Check sheet for the modelled part. Datum: model origin and axes. Units: mm. A direction names the side the tool comes from. Coordinates: 2 decimals unless noted, no trailing zeros. Order: outer loops, then holes, each group sorted by start corner. A loop starts at its lowest first (then second) coordinate and runs counter-clockwise, first axis right, second up.
from build123d import *

# Parameters (mm, degrees)
F1_DEPTH     = 113.387234509
F3_DEPTH     = 464.7335410118
F5_DEPTH     = 66.4555206895
F6_R         = 30.48
F8_DEPTH     = 322.3102986813
F10_DEPTH    = 342.2025442123
F12_DEPTH    = 991.1689758301
F13_T4_DEPTH = 1291.048119331


# Not quite as in the source:
# - a fillet or chamfer that OpenCascade refuses, or shapes differently, is made with other operations: its cross-section is extruded or revolved along the edge and cut away or added


with BuildPart() as f1:
    # F0 (on Front) → F1 (new body)
    with BuildSketch(Plane.XZ):
        Polygon((-915.6464338303, -243.6540126801), (1070.1038837433, -243.6540126801), (312.4090433121, 163.7299656868), (-915.6464338303, -88.1789922714), align=None)
    extrude(amount=-F1_DEPTH)

    # F2 (on face) → F3 (join)
    with BuildSketch(Plane.XZ):
        Polygon((-516.0537958145, -243.6540126801), (938.1332397461, -243.6540126801), (502.8445720673, -57.6961040497), (-296.7971563339, -57.6961040497), (-296.7971563339, -109.2859506607), (-403.2011032104, -109.2859506607), (-403.2011032104, -167.32442379), (-516.0537958145, -167.32442379), align=None)
    extrude(amount=F3_DEPTH)

    # F4 (on face) → F5 (join)
    with BuildSketch(Plane.XZ.offset(464.7335410118)):
        Polygon((528.1958580017, -243.6540126801), (938.1332397461, -243.6540126801), (398.7933658153, -13.2448096747), (-296.7971563339, -13.2448096747), (-877.5278925896, -136.8308067322), (-877.5278925896, -243.4085607529), align=None)
    extrude(amount=F5_DEPTH)

    # F6
    f6_edges = [f1.edges().sort_by_distance(p)[0] for p in [
        (50.998105, -464.733541, -13.24481),
        (50.998105, -531.189062, -13.24481),
        (-587.162524, -531.189062, -75.037808),
        (-587.162524, -464.733541, -75.037808),
    ]]
    fillet(f6_edges, radius=F6_R)

    # F7 (on face) → F8 (join)
    with BuildSketch(Plane.XZ.offset(531.1890617013)):
        Polygon((-543.689250946, -243.4668519626), (938.1332397461, -243.6540126801), (598.4011143715, -98.5184274462), (-393.8011527061, -98.5184274462), (-393.8011527061, -143.1138366461), (-464.6941423416, -143.1138366461), (-464.6941423416, -195.7771629095), (-543.689250946, -195.7771629095), align=None)
    extrude(amount=F8_DEPTH)

    # F9 (on face) → F10 (join)
    with BuildSketch(Plane.XZ.offset(853.4993603826)):
        Polygon((938.1332397461, -243.6540126801), (598.4011143715, -98.5184274462), (598.4011143715, -243.6111030139), align=None)
    extrude(amount=F10_DEPTH)

    # F11 (on face) → F12 (join)
    with BuildSketch(Plane(origin=(598.4011143715, 0, 0), x_dir=(0, -1, 0), z_dir=(-1, 0, 0))):
        Polygon((853.4993603826, -98.5184274462), (853.4993603826, -243.6111030139), (1195.7019045949, -243.6111030139), align=None)
    extrude(amount=F12_DEPTH)

    # F13: chamfer of 254 x 368.3 on 1 edges, made by hand


with BuildPart() as f13_tool2:
    # F13_s3 → F13_t4 (new body)
    with BuildSketch(Plane.XZ.offset(853.4993603826)):
        Polygon((937.089450141, -243.2080995506), (598.4011143715, -352.5184274462), (598.4011143715, -98.5184274462), align=None)
    extrude(amount=F13_T4_DEPTH)

    split(bisect_by=Plane(origin=(0, -94.6492992071, 223.2313303883), x_dir=(1, 0, 0), z_dir=(0, -0.3903579472, 0.9206631703)), keep=Keep.TOP)


with BuildPart() as f1_1:
    add(f1.part)

    # F13_t1: cut F13_tool2
    add(f13_tool2.part, mode=Mode.SUBTRACT)


solid = f1_1.part
(1) Cross-section at A-A (y = -654). Enter the section's corners in (x, z), and give its area (3 significant figures).
Filled in:
outline: (-543.69, -243.47) - (938.13, -243.65) - (598.4, -98.52) - (-393.8, -98.52) - (-393.8, -143.11) - (-464.69, -143.11) - (-464.69, -195.78) - (-543.69, -195.78) - close
area: 179,000 mm2
(2) Cross-section at D-D (z = -217). Enter the section's corners in (x, y).
Filled in:
outline: (-915.65, 0) - (-516.05, 0) - (-516.05, -464.73) - (-877.53, -464.73) - (-877.53, -531.19) - (-543.69, -531.19) - (-543.69, -853.5) - (-392.77, -853.5) - (-392.77, -1132.94) - (875.74, -1132.94) - (875.74, 0) - (1020.53, 0) - (1020.53, 113.39) - (-915.65, 113.39) - close
(3) Go/stop test with flat-tipped pins: P1, Ø6, axis at y = -147.5, z = -153.5, coming from the -X side; P2, Ø12, axis at y = -70.5, z = -70.5, coming from the -X side; P3, Ø5, axis at x = 36, z = 98, coming from the -Y side. Record where each tip stops, or that it passes through.
Filled in:
P1: stops at x = -403.2
P2: stops at x = -296.8
P3: stops at y = 0
(4) Tool access check on faces 5 (the flat face through (-349, -229, -109.286)), 6 (the flat face through (-877.528, -497, -189)), 7 (the flat face through (732.165, -456.625, -155.663)), 8 (the flat face through (-516.054, -229, -205)), 9 (the flat face through (-583.097, -497.923, -74.173)). Record the directions out of +Z, -Z, +X, -X, +Y, -Y that give a thin tool (end or side, any length) a straight path to the whole face; none if there is none.
Filled in:
face 5: +Z, -X
face 6: +Z, -Z, -X, -Y
face 7: +Z, +X, -Y
face 8: +Z, -Z, -X
face 9: +Z, -X, -Y
(5) Thickness scan on probe 1 along Y at (x, z) = (347, -43); probe 2 along Z at (x, y) = (-113.5, -236); probe 3 along Z at (x, y) = (-510, -538). Record the ranges inside material, lowest first.
Filled in:
probe 1: y = -531.18 to -464.74, 0 to 113.39
probe 2: z = -243.65 to -57.7
probe 3: z = -243.47 to -195.78
(6) Release check for a two-part mould opening along Y. For faces 1 (the flat face through (-459, -229, -167.324)), 2 (the flat face through (-392.768, -946, -202)), 3 (the flat face through (63, 113.387, -82)), 4 (the flat face through (-296.797, -229, -83)) record: +Y half, -Y half, draft (parallel to the pull), parting line (faces both ways), or undercut.
Filled in:
face 1: undercut
face 2: draft
face 3: +Y half
face 4: undercut
(7) Cross-section at C-C (y = -178.5). Enter the section's corners in (x, z), and give its area (3 significant figures).
Filled in:
outline: (-516.05, -243.65) - (938.13, -243.65) - (502.84, -57.7) - (-296.8, -57.7) - (-296.8, -109.29) - (-403.2, -109.29) - (-403.2, -167.32) - (-516.05, -167.32) - close
area: 212,000 mm2
